```python
from build123d import *

# Parameters (mm, degrees)
SKETCH1_R           = 1.5875
SKETCH1_R_2         = 1.778
SKETCH1_R_3         = 2.54
SKETCH1_R_4         = 5.08
BOSS_EXTRUDE1_DEPTH = 6.35


with BuildPart() as part:
    # Sketch1 → Boss-Extrude1 (new body)
    with BuildSketch(Plane.XY):
        Polygon((249.789850187, 150.240558714), (314.789850187, 150.240558714), (314.789850187, -49.759441286), (249.789850187, -49.759441286), (249.789850187, -19.759441286), (179.789850187, -19.759441286), (179.789850187, -49.759441286), (114.789850187, -49.759441286), (114.789850187, 150.240558714), (179.789850187, 150.240558714), (179.789850187, 120.240558714), (249.789850187, 120.240558714), align=None)
        with Locations((140.189850187, -8.179441286)):
            Circle(SKETCH1_R, mode=Mode.SUBTRACT)
        with Locations((122.409850187, 62.940558714)):
            Circle(SKETCH1_R_2, mode=Mode.SUBTRACT)
        with Locations((122.409850187, 37.540558714)):
            Circle(SKETCH1_R_2, mode=Mode.SUBTRACT)
        with Locations((147.809850187, 37.540558714)):
            Circle(SKETCH1_R_2, mode=Mode.SUBTRACT)
        with Locations((140.189850187, 108.660558714)):
            Circle(SKETCH1_R, mode=Mode.SUBTRACT)
        with Locations((147.809850187, 62.940558714)):
            Circle(SKETCH1_R_2, mode=Mode.SUBTRACT)
        with Locations((281.769850187, 62.940558714)):
            Circle(SKETCH1_R_2, mode=Mode.SUBTRACT)
        with Locations((307.169850187, 62.940558714)):
            Circle(SKETCH1_R_2, mode=Mode.SUBTRACT)
        with Locations((281.769850187, 37.540558714)):
            Circle(SKETCH1_R_2, mode=Mode.SUBTRACT)
        with Locations((307.169850187, 37.540558714)):
            Circle(SKETCH1_R_2, mode=Mode.SUBTRACT)
        with Locations((121.139850187, 143.890558714)):
            Circle(SKETCH1_R_3, mode=Mode.SUBTRACT)
        with Locations((140.189850187, 89.597220113)):
            Circle(SKETCH1_R_3, mode=Mode.SUBTRACT)
        with Locations((203.689850187, 89.597220113)):
            Circle(SKETCH1_R_3, mode=Mode.SUBTRACT)
        with Locations((191.294850187, 11.990558714)):
            Circle(SKETCH1_R_2, mode=Mode.SUBTRACT)
        with Locations((197.136850187, 11.990558714)):
            Circle(SKETCH1_R_2, mode=Mode.SUBTRACT)
        with Locations((191.294850187, 5.640558714)):
            Circle(SKETCH1_R_2, mode=Mode.SUBTRACT)
        with Locations((197.136850187, 5.640558714)):
            Circle(SKETCH1_R_2, mode=Mode.SUBTRACT)
        with Locations((191.294850187, 94.840558714)):
            Circle(SKETCH1_R_2, mode=Mode.SUBTRACT)
        with Locations((191.294850187, 88.490558714)):
            Circle(SKETCH1_R_2, mode=Mode.SUBTRACT)
        with Locations((197.136850187, 88.490558714)):
            Circle(SKETCH1_R_2, mode=Mode.SUBTRACT)
        with Locations((197.136850187, 94.840558714)):
            Circle(SKETCH1_R_2, mode=Mode.SUBTRACT)
        with Locations((166.529850187, 74.370558714)):
            Circle(SKETCH1_R_3, mode=Mode.SUBTRACT)
        with Locations((241.459850187, 74.370558714)):
            Circle(SKETCH1_R_3, mode=Mode.SUBTRACT)
        with Locations((166.529850187, 26.110558714)):
            Circle(SKETCH1_R_3, mode=Mode.SUBTRACT)
        with Locations((247.809850187, 26.110558714)):
            Circle(SKETCH1_R_3, mode=Mode.SUBTRACT)
        with Locations((121.139850187, -43.409441286)):
            Circle(SKETCH1_R_3, mode=Mode.SUBTRACT)
        with Locations((308.439850187, -43.409441286)):
            Circle(SKETCH1_R_3, mode=Mode.SUBTRACT)
        with Locations((308.439850187, 143.890558714)):
            Circle(SKETCH1_R_3, mode=Mode.SUBTRACT)
        with Locations((165.076665974, 113.740558714)):
            Circle(SKETCH1_R_4, mode=Mode.SUBTRACT)
        with Locations((165.076665974, -13.259441286)):
            Circle(SKETCH1_R_4, mode=Mode.SUBTRACT)
        with BuildLine():
            Line((135.109850187, 19.760558714), (172.953168155, 19.760558714))
            ThreePointArc((172.953168155, 19.760558714), (181.843168155, 10.870558714), (172.953168155, 1.980558714))
            Line((172.953168155, 1.980558714), (135.109850187, 1.980558714))
            ThreePointArc((135.109850187, 1.980558714), (126.219850187, 10.870558714), (135.109850187, 19.760558714))
        make_face(mode=Mode.SUBTRACT)
        with BuildLine():
            Line((218.269850187, 98.500558714), (294.469850187, 98.500558714))
            ThreePointArc((294.469850187, 98.500558714), (303.359850187, 89.610558714), (294.469850187, 80.720558714))
            Line((294.469850187, 80.720558714), (218.269850187, 80.720558714))
            ThreePointArc((218.269850187, 80.720558714), (209.379850187, 89.610558714), (218.269850187, 98.500558714))
        make_face(mode=Mode.SUBTRACT)
        with BuildLine():
            Line((214.789850187, 1.980558714), (294.469850187, 1.980558714))
            ThreePointArc((294.469850187, 1.980558714), (303.359850187, 10.870558714), (294.469850187, 19.760558714))
            Line((294.469850187, 19.760558714), (214.789850187, 19.760558714))
            ThreePointArc((214.789850187, 19.760558714), (205.899850187, 10.870558714), (214.789850187, 1.980558714))
        make_face(mode=Mode.SUBTRACT)
    extrude(amount=BOSS_EXTRUDE1_DEPTH)


solid = part.part
```
Check sheet for the modelled part. Datum: model origin and axes. Units: mm. A direction names the side the tool comes from. Give positions to 0.01 mm unless a question says otherwise; leave off trailing zeros. Order: outer loops, then holes, each group sorted by start corner. A loop starts at its lowest first (then second) coordinate and runs counter-clockwise, first axis right, second up. Notation, with made-up numbers: (27.25, 10.5) -> (57.25, 10.5) arc R30 ccw to (57.25, 43.5) -> close; hole circle Ø4 at (42.25, 17). An arc over 180 degrees is marked (long way). Use CSV: the item, a comma, the result in double quotes. Start each with the question number.
1) Mould release check, pull along X, two halves, no side actions. Record for faces 5 (the face through (147, 150.241, 3)), 6 (the face through (255, 19.761, 3)): released by +X, released by -X, zero draft, split by the parting line, or undercut.
2) Material ranges on line 1 (Y direction, x = 219, z = 3.75); line 2 (Y direction, x = 275.5, z = 5); line 3 (X direction, y = -23.5, z = 3.5), recorded low to high. Write a range as from..to.
3) Go/stop test with flat-tipped pins: P1, Ø3, axis at x = 203.69, y = 89.6, coming from the -Z side; P2, Ø3, axis at x = 223, z = 4.5, coming from the +Y side. Record where each tip stops, or that it passes through.
4) Sectioned sample at D-D, the plane z = 3.75. Give the number of separate pieces and of enclosed holes in the cut face, plus the area to 3 significant figures.
5) Sectioned sample at B-B, the plane y = -31.5. Record the boundary of the cut face in (x, z).
6) Set-up check for faces 1 (the face through (249.79, -35, 3)), 2 (the face through (214, 120.241, 3)), 3 (the face through (216, 52, 0)), 4 (the face through (154, 19.761, 3)): record each of +Z, -Z, +X, -X, +Y, -Y from which the full face is reachable in a straight line by a thin tool's end or side.
7) Sectioned sample at C-C, the plane x = 223. Record the boundary of the cut face in (y, z).
8) Sectioned sample at A-A, the plane x = 275. Record the boundary of the cut face in (y, z).
Recorded:
1,face 5,"zero draft"
1,face 6,"undercut"
2,line 1,"-19.76..1.98, 19.76..80.72, 98.5..120.24"
2,line 2,"-49.76..1.98, 19.76..80.72, 98.5..150.24"
2,line 3,"114.79..179.79, 249.79..314.79"
3,P1,"through"
3,P2,"y = 120.24"
4,separate pieces,"1"
4,enclosed holes,"33"
4,area,"31,100 mm2"
5,outline,"(114.79, 0) -> (179.79, 0) -> (179.79, 6.35) -> (114.79, 6.35) -> close; (249.79, 0) -> (314.79, 0) -> (314.79, 6.35) -> (249.79, 6.35) -> close"
6,face 1,"+Z, -Z, -Y"
6,face 2,"+Z, -Z, +Y"
6,face 3,"-Z, +X, -X, +Y, -Y"
6,face 4,"+Z, -Z"
7,outline,"(-19.76, 0) -> (1.98, 0) -> (1.98, 6.35) -> (-19.76, 6.35) -> close; (19.76, 0) -> (80.72, 0) -> (80.72, 6.35) -> (19.76, 6.35) -> close; (98.5, 0) -> (120.24, 0) -> (120.24, 6.35) -> (98.5, 6.35) -> close"
8,outline,"(-49.76, 0) -> (1.98, 0) -> (1.98, 6.35) -> (-49.76, 6.35) -> close; (19.76, 0) -> (80.72, 0) -> (80.72, 6.35) -> (19.76, 6.35) -> close; (98.5, 0) -> (150.24, 0) -> (150.24, 6.35) -> (98.5, 6.35) -> close"
